Work out the finished part from the listing and answer in its coordinate system (mm). Face numbers are marked on the shaded views. A direction names the side the tool comes from. Round coordinates to 2 decimals unless told otherwise and drop trailing zeros. Write each loop counter-clockwise with the first axis right and the second up, starting at its lowest first coordinate (ties: lowest second). Pieces come first, ordered by that corner, then holes. Notation, with made-up numbers: M 39,38 L 67,38 A15 cw 67,61 Z; hole C 44.5,53 d11. An arc over 180 degrees is marked long. Answer in a Markdown table with one row per item.
```python
from build123d import *

# Parameters (mm, degrees)
SKETCH1_W           = 20
SKETCH1_H           = 10
BOSS_EXTRUDE1_DEPTH = 5
SKETCH2_W           = 17.6
SKETCH2_H           = 2.6
BOSS_EXTRUDE2_DEPTH = 4
FILLET1_R           = 0.7
SKETCH3_W           = 20
SKETCH3_H           = 7.5
BOSS_EXTRUDE3_DEPTH = 17
SKETCH4_R           = 2.1
BOSS_EXTRUDE4_DEPTH = 6.5


with BuildPart() as part:
    # Sketch1 → Boss-Extrude1 (new body)
    with BuildSketch(Plane(origin=(0, 0, 0), x_dir=(1, 0, 0), z_dir=(0, 1, 0))):
        Rectangle(SKETCH1_W, SKETCH1_H)
    extrude(amount=BOSS_EXTRUDE1_DEPTH)

    # Sketch2 → Boss-Extrude2 (add)
    with BuildSketch(Plane(origin=(0, 0, -5), x_dir=(-1, 0, 0), z_dir=(0, 0, -1))):
        with Locations((0, 2.5)):
            Rectangle(SKETCH2_W, SKETCH2_H)
    extrude(amount=BOSS_EXTRUDE2_DEPTH)

    # Fillet1
    fillet1_edges = [part.edges().sort_by_distance(p)[0] for p in [
        (-8.8, 1.2, -7),
        (-8.8, 3.8, -7),
        (8.8, 3.8, -7),
        (8.8, 1.2, -7),
    ]]
    fillet(fillet1_edges, radius=FILLET1_R)

    # Sketch3 → Boss-Extrude3 (add)
    with BuildSketch(Plane(origin=(0, 5, 0), x_dir=(1, 0, 0), z_dir=(0, 1, 0))):
        with Locations((0, -1.25)):
            Rectangle(SKETCH3_W, SKETCH3_H)
    extrude(amount=BOSS_EXTRUDE3_DEPTH)

    # Sketch4 → Boss-Extrude4 (add)
    with BuildSketch(Plane(origin=(0, 0, -2.5), x_dir=(-1, 0, 0), z_dir=(0, 0, -1))):
        with Locations((0, 12)):
            Circle(SKETCH4_R)
    extrude(amount=BOSS_EXTRUDE4_DEPTH)


solid = part.part
```
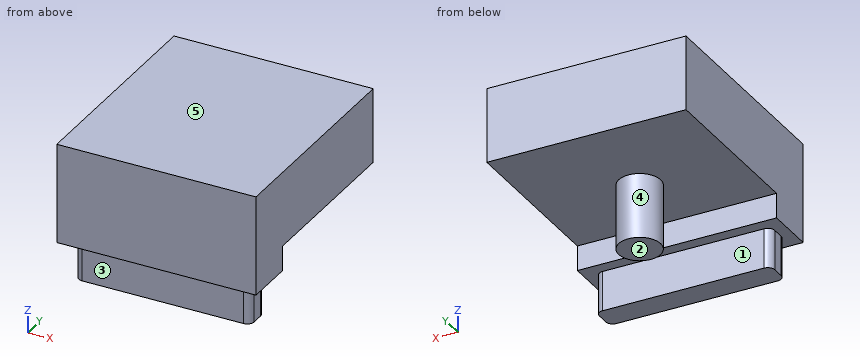
1. The part is cut by section C-C (y = 12). Determine the outline of the cut face in (x, z), plus the area to 3 significant figures.
Calculated:
| item | result |
|---|---|
| outline | M -10,-2.5 L -2.1,-2.5 L -2.1,-9 L 2.1,-9 L 2.1,-2.5 L 10,-2.5 L 10,5 L -10,5 Z |
| area | 177 mm² |
2. The part is cut by section A-A (x = 5.25). Determine the outline of the cut face in (y, z), plus the area to 3 significant figures.
Calculated:
| item | result |
|---|---|
| outline | M 0,-5 L 1.2,-5 L 1.2,-9 L 3.8,-9 L 3.8,-5 L 5,-5 L 5,-2.5 L 22,-2.5 L 22,5 L 0,5 Z |
| area | 188 mm² |
3. Determine the mould class of the marked faces 3, 4 and 5 for opening direction Y: released by +Y, released by -Y, zero draft, split by the parting line, or undercut.
Calculated:
| item | result |
|---|---|
| face 3 | released by -Y |
| face 4 | undercut |
| face 5 | zero draft |
4. Given pin 1 (2 mm diameter, centred on x = 1, z = -7, fed in from -Y); pin 2 (5 mm diameter, centred on x = -1, z = -5.5, fed in from +Y); pin 3 (0.6 mm diameter, centred on y = 2.5, z = -7, fed in from +X), each flat-ended and moving along its own axis, determine where each tip first touches the part or whether it passes through.
Calculated:
| item | result |
|---|---|
| pin 1 | stops at y = 1.2 |
| pin 2 | stops at y = 14.1 |
| pin 3 | stops at x = 8.8 |
5. A tool of negligible diameter and unlimited length cuts with its end or side. For the marked faces 1 and 2, from which of +Z, -Z, +X, -X, +Y, -Y can it reach the whole face along a straight path? Write none if from no direction.
Calculated:
| item | result |
|---|---|
| face 1 | -Z, +X, -X |
| face 2 | -Z, +X, -X, +Y, -Y |
6. Consider line 1 along Z through (x, y) = (2, 17.75); line 2 along Y through (x, z) = (5, -3); line 3 along Y through (x, z) = (-7.75, -5.5). Determine where each line is inside the solid, lowest interval first. Write a range as from..to.
Calculated:
| item | result |
|---|---|
| line 1 | z = -2.5..5 |
| line 2 | y = 0..5 |
| line 3 | y = 1.2..3.8 |
7. The part is cut by section B-B (z = -4.5). Determine the outline of the cut face in (x, y).
Calculated:
| item | result |
|---|---|
| outline | M -10,0 L 10,0 L 10,5 L -10,5 Z; C 0,12 d4.2 |
8. The part is cut by section D-D (x = 0). Determine the outline of the cut face in (y, z), plus the area to 3 significant figures.
Calculated:
| item | result |
|---|---|
| outline | M 0,-5 L 1.2,-5 L 1.2,-9 L 3.8,-9 L 3.8,-5 L 5,-5 L 5,-2.5 L 9.9,-2.5 L 9.9,-9 L 14.1,-9 L 14.1,-2.5 L 22,-2.5 L 22,5 L 0,5 Z |
| area | 215 mm² |
